from build123d import *

# Parameters (mm, degrees)
F0_W          = 12.7
F0_H          = 12.7
F1_DEPTH      = 19.05
F2_R          = 1.5875
F3_DEPTH      = 25.4
F4_R          = 1.5875
F5_DEPTH      = 6.351
F5_DEPTH_BACK = 6.351
F6_R          = 3.175
F7_DEPTH      = 12.7
F8_R          = 1.905
F9_SIZE       = 0.254


with BuildPart() as f1:
    # F0 (on Top) → F1 (new body)
    with BuildSketch(Plane.XY):
        Rectangle(F0_W, F0_H)
    extrude(amount=F1_DEPTH)

    # F2 (on face) → F3 (cut)
    with BuildSketch(Plane.XZ.offset(6.35)):
        with Locations((0, 6.35)):
            Circle(F2_R)
    extrude(amount=-F3_DEPTH, mode=Mode.SUBTRACT)

    # F4 (on Right) → F5 (cut, two sides)
    with BuildSketch(Plane.YZ) as f5_sk:
        with Locations((0, 6.35)):
            Circle(F4_R)
    extrude(amount=-F5_DEPTH, mode=Mode.SUBTRACT)
    extrude(f5_sk.sketch, amount=F5_DEPTH_BACK, mode=Mode.SUBTRACT)

    # F6 (on face) → F7 (cut)
    with BuildSketch(Plane.XY.offset(19.05)):
        Circle(F6_R)
    extrude(amount=-F7_DEPTH, mode=Mode.SUBTRACT)

    # F8
    f8_edges = [f1.edges().sort_by_distance(p)[0] for p in [
        (-6.35, 0, 19.05),
        (0, -6.35, 19.05),
        (6.35, 0, 19.05),
        (0, 6.35, 19.05),
        (6.35, -6.35, 9.525),
        (6.35, 6.35, 9.525),
        (-6.35, -6.35, 9.525),
        (-6.35, 6.35, 9.525),
        (-6.35, 0, 0),
        (0, -6.35, 0),
        (6.35, 0, 0),
        (0, 6.35, 0),
    ]]
    fillet(f8_edges, radius=F8_R)

    # F9
    f9_edges = [f1.edges().sort_by_distance(p)[0] for p in [
        (6.35, -1.5875, 6.35),
        (-3.175, 0, 19.05),
        (-1.5875, 6.35, 6.35),
        (-6.35, -1.5875, 6.35),
        (-1.5875, -6.35, 6.35),
    ]]
    chamfer(f9_edges, length=F9_SIZE)


solid = f1.part
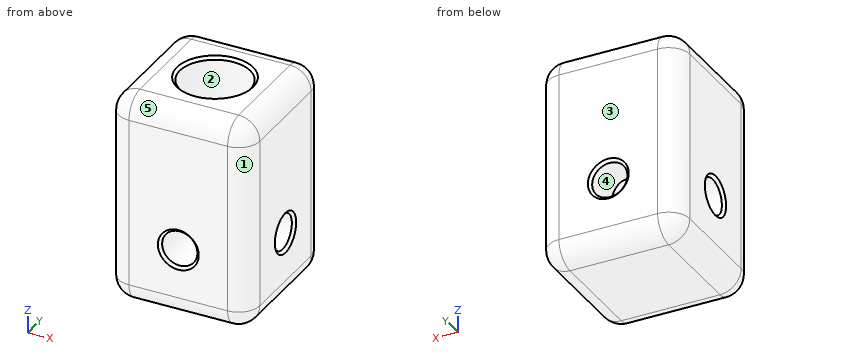
Could you check a few things on this model? Use its own coordinates, in mm. Face numbers are marked on the shaded views. A direction names the side the tool comes from. Give positions to 0.01 mm unless a question says otherwise; leave off trailing zeros. Write each loop counter-clockwise with the first axis right and the second up, starting at its lowest first coordinate (ties: lowest second). Pieces come first, ordered by that corner, then holes. Notation, with made-up numbers: (17.25, -7.75) - (65.25, -7.75) arc R23 cw to (65.25, 16.25) - close; hole circle Ø3 at (56, 82). An arc over 180 degrees is marked (long way). Use CSV: the item, a comma, the result in double quotes. Start each with the question number.
Item 1: For the marked faces 1 and 2, which set-ups out of +Z, -Z, +X, -X, +Y, -Y let a thin tool reach every point of the face, with its end or its side?
Item 2: I want a section at B-B, the plane x = 0.5. Give the number of separate pieces and of enclosed holes in the cut face, then the cut area to 3 significant figures.
Item 3: I want a section at A-A, the plane z = 16.5. Please give me the cut outline in (x, y) (3 decimals).
Item 4: If I drill on line 1 along Z through (x, y) = (-4, 0); line 2 along X through (y, z) = (0, 12.75) (3 decimals); line 3 along X through (y, z) = (2.75, 15.75), over which ranges is the centre line in solid material (lowest first)?
Item 5: I'm going to push flat-ended pins straight in: pin 1 (3 mm diameter, centred on x = 0, z = 6.35, fed in from +Y); pin 2 (3.5 mm diameter, centred on y = 0, z = 6.35, fed in from -X); pin 3 (0.6 mm diameter, centred on x = 2, y = -2, fed in from +Z); pin 4 (0.9 mm diameter, centred on x = -2, y = 2, fed in from +Z). Where does each tip first touch, or does it pass through?
Item 6: If we mould it in two halves opening along Z, with no side actions, what happens to the marked faces 3, 4 and 5? For each: pulls with the +Z half, pulls with the -Z half, needs draft (parallel to the pull), parting line crosses it, or undercut.
Findings:
1,face 1,"+Z, -Z, +X, -Y"
1,face 2,"+Z"
2,separate pieces,"3"
2,enclosed holes,"0"
2,area,"130 mm2"
3,outline,"(-6.35, -4.445) arc R1.905 ccw to (-4.445, -6.35) - (4.445, -6.35) arc R1.905 ccw to (6.35, -4.445) - (6.35, 4.445) arc R1.905 ccw to (4.445, 6.35) - (-4.445, 6.35) arc R1.905 ccw to (-6.35, 4.445) - close; hole circle Ø6.35 at (0, 0)"
4,line 1,"z = 0 to 4.76, 7.94 to 19.05"
4,line 2,"x = -6.35 to -3.175, 3.175 to 6.35"
4,line 3,"x = -6.35 to -1.59, 1.59 to 6.35"
5,pin 1,"passes through"
5,pin 2,"stops at x = -6.26"
5,pin 3,"stops at z = 6.35"
5,pin 4,"stops at z = 18.9"
6,face 3,"needs draft"
6,face 4,"undercut"
6,face 5,"pulls with the +Z half"
